The model under review builds one solid part; all positions refer to its coordinate system, in mm. A direction names the side the tool comes from. Coordinates: 2 decimals unless noted, no trailing zeros. Write each loop counter-clockwise with the first axis right and the second up, starting at its lowest first coordinate (ties: lowest second). Pieces come first, ordered by that corner, then holes. Notation, with made-up numbers: (84.5, 3.5) - (97.5, 3.5) arc R7 cw to (97.5, 15.5) - close; hole circle Ø2 at (-2.5, 35). An arc over 180 degrees is marked (long way). Put each result on its own line as item: value.
from build123d import *

# Parameters (mm, degrees)
BOSS_EXTRUDE1_DEPTH  = 6
M3_CLEARANCE_HOLE1_D = 3.4


with BuildPart() as part:
    # Sketch1 → Boss-Extrude1 (new body)
    with BuildSketch(Plane.XY):
        Polygon((120, 72), (150, 72), (150, -72), (120, -72), (120, -99.5), (-120, -99.5), (-120, -72), (-150, -72), (-150, 72), (-120, 72), (-120, 99.5), (120, 99.5), align=None)
    extrude(amount=BOSS_EXTRUDE1_DEPTH)

    # M3 Clearance Hole1 (through all)
    with Locations(Plane(origin=(-60, 40, 6), x_dir=(1, 0, 0), z_dir=(0, 0, 1))):
        with Locations((0, 0), (0, -80), (120, -80), (120, 0)):
            Hole(M3_CLEARANCE_HOLE1_D / 2)


solid = part.part
1. Consider section B-B on y = 86.5. State the section outline as (x, z) points.
Determined:
outline: (-120, 0) - (120, 0) - (120, 6) - (-120, 6) - close
2. For pin 1 Ø3 at (y, z) = (-90.5, 2) entering from -X; pin 2 Ø3 at (x, z) = (-129, 4) entering from +Y; pin 3 Ø3 at (x, y) = (60, -40) entering from -Z; pin 4 Ø1.5 at (y, z) = (-74.5, 5) entering from +X, all flat-tipped, find the tip position at first contact; note any pin that passes through.
Determined:
pin 1: stops at x = -120
pin 2: stops at y = 72
pin 3: passes through
pin 4: stops at x = 120
3. To check wall thickness, follow probe 1 along Y at (x, z) = (60, 2.25); probe 2 along X at (y, z) = (-80, 3.5). State the ranges of each line that lie inside material, in increasing order.
Determined:
probe 1: y = -99.5 to -41.7, -38.3 to 38.3, 41.7 to 99.5
probe 2: x = -120 to 120
4. Consider section A-A on z = 4.1. State the section outline as (x, y) points, plus the area to 3 significant figures.
Determined:
outline: (-150, -72) - (-120, -72) - (-120, -99.5) - (120, -99.5) - (120, -72) - (150, -72) - (150, 72) - (120, 72) - (120, 99.5) - (-120, 99.5) - (-120, 72) - (-150, 72) - close; hole circle Ø3.4 at (-60, -40); hole circle Ø3.4 at (-60, 40); hole circle Ø3.4 at (60, -40); hole circle Ø3.4 at (60, 40)
area: 56,400 mm^2
5. Machinability: for faces 1 (the flat face through (120, 86, 3)), 2 (the flat face through (-135, -72, 3)), 3 (the flat face through (-120, 86, 3)), 4 (the flat face through (120, -86, 3)), which of the approach directions +Z, -Z, +X, -X, +Y, -Y give a long, thin tool a straight path to every point of the face, cutting with its end or side? Answer none if there is none.
Determined:
face 1: +Z, -Z, +X, +Y
face 2: +Z, -Z, -X, -Y
face 3: +Z, -Z, -X, +Y
face 4: +Z, -Z, +X, -Y
